```python
from build123d import *

# Parameters (mm, degrees)
F2_R      = 20.3245328948
F1_R      = 39.0974153035
F4_R      = 21.0995662857
F5_R      = 2.5836298092
F3_FACE_R = 39.0974153035
F10_R     = 14.6545023438
F12_R     = 152.4
F14_DEPTH = 12.7
F15_DEPTH = 12.7
F16_R     = 3.4719949567
F16_R_2   = 4.7718005113
F17_DEPTH = 25.4


with BuildPart() as f3:
    # F2 (on offset) → F3 section 0
    with BuildSketch(Plane.XY.offset(101.6)):
        Circle(F2_R)
    # F1 (on Top) → F3 section 1
    with BuildSketch(Plane.XY):
        Circle(F1_R)
    loft()

    # F4
    f4_edges = [f3.edges().sort_by_distance(p)[0] for p in [
        (-20.324533, 0, 101.6),
    ]]
    fillet(f4_edges, radius=F4_R)

    # F5 (on offset) → F8 section 0
    with BuildSketch(Plane.XY.offset(101.6), mode=Mode.PRIVATE) as f8_s0:
        Circle(F5_R)
    loft([f8_s0.sketch, Vertex(0, 0, 208.026)])

    # F3_face (on face) → F11 section 0
    with BuildSketch(Plane(origin=(0, 0, 0), x_dir=(1, 0, 0), z_dir=(0, 0, -1))):
        Circle(F3_FACE_R)
    # F10 (on offset) → F11 section 1
    with BuildSketch(Plane.XY.offset(-167.64)):
        Circle(F10_R)
    loft()

    # F12
    f12_edges = [f3.edges().sort_by_distance(p)[0] for p in [
        (-39.097415, 0, 0),
    ]]
    fillet(f12_edges, radius=F12_R)

    # F13 (on Right) → F14 (join)
    with BuildSketch(Plane.YZ):
        Polygon((14.7928362712, -167.672470212), (-14.6080739796, -167.5585210323), (-19.3942692131, -179.0681779385), (0, -172.4586635828), (17.5278056413, -182.3729276657), align=None)
    extrude(amount=F14_DEPTH)

    # F13 (on Right) → F15 (join)
    with BuildSketch(Plane.YZ):
        Polygon((14.7928362712, -167.672470212), (-14.6080739796, -167.5585210323), (-19.3942692131, -179.0681779385), (0, -172.4586635828), (17.5278056413, -182.3729276657), align=None)
    extrude(amount=-F15_DEPTH)

    # F16 (on Right) → F17 (cut)
    with BuildSketch(Plane.YZ):
        with Locations((22.7732714266, 55.7852126658)):
            Circle(F16_R)
        with Locations((-19.15024966, 54.7500625253)):
            Circle(F16_R_2)
    extrude(amount=-F17_DEPTH, mode=Mode.SUBTRACT)


solid = f3.part
```
The listing builds one solid part. Answer for the finished solid, in the listing's coordinates (mm). A direction names the side the tool comes from. Coordinates: 2 decimals unless noted, no trailing zeros. Write each loop counter-clockwise with the first axis right and the second up, starting at its lowest first coordinate (ties: lowest second). Pieces come first, ordered by that corner, then holes.
Q1. Given P1, Ø8, axis at y = -25, z = -39, coming from the +X side; P2, Ø1.5, axis at y = 2, z = -133.5, coming from the -X side; P3, Ø5, axis at x = -1.5, y = -1.5, coming from the +Z side; P4, Ø7.5, axis at y = 24, z = 54.5, coming from the -X side, each flat-ended and moving along its own axis, determine where each tip first touches the part or whether it passes through.
Returned:
P1: stops at x = 26.07
P2: stops at x = -19.66
P3: stops at z = 208.03
P4: stops at x = -20.9
Q2. Which of the six approach directions +Z, -Z, +X, -X, +Y, -Y give full straight-line access (tool end or side, diameter ignored) to faces 1 (the flat face through (0, 23, 56)), 2 (the conical face through (23.763, -7.483, -97.278)), 3 (the flat face through (0.2, -9.8, -175.8)), 4 (the flat face through (0.18, 16.18, -175.13))?
Returned:
face 1: -X
face 2: none
face 3: -Z, +X, -X
face 4: +X, -X, +Y
Q3. Find the intervals of material crossed by line 1 along Z through (x, y) = (-10, 3); line 2 along X through (y, z) = (-23.5, 24.5); line 3 along Y through (x, z) = (-12, -16), in increasing order.
Returned:
line 1: z = -174.16 to 100.16
line 2: x = -25.35 to 25.35
line 3: y = -34.47 to 34.47
Q4. Section B-B, the plane x = -7 is taken. Give the number of separate pieces and of enclosed holes in the cut face, then the cut area to 3 significant figures.
Returned:
separate pieces: 1
enclosed holes: 2
area: 14,500 mm2
Q5. Section A-A, the plane z = 162.5 is taken. Write down the section's boundary in (x, y).
Returned:
outline: circle Ø2.21 at (0, 0)
